from build123d import *

# Parameters (mm, degrees)
BOSS_EXTRUDE1_DEPTH = 5.772427301
SKETCH2_W           = 10.772427301
SKETCH2_H           = 33
BOSS_EXTRUDE2_DEPTH = 1
CUT_EXTRUDE1_DEPTH  = 2
SKETCH16_W          = 10.772427301
SKETCH16_H          = 1
BOSS_EXTRUDE4_DEPTH = 11
CUT_EXTRUDE2_REACH  = 24.797
SKETCH26_W          = 5
SKETCH26_H          = 10.722198916
CUT_EXTRUDE3_DEPTH  = 24.875254024
SKETCH13_W          = 3.772427301
SKETCH13_H          = 2.348567359
CUT_EXTRUDE4_DEPTH  = 1
SKETCH27_W          = 1
SKETCH27_H          = 12
BOSS_EXTRUDE5_DEPTH = 2.235
SKETCH28_W          = 1
SKETCH28_H          = 12
BOSS_EXTRUDE6_DEPTH = 2.235


with BuildPart() as part:
    # Sketch1 → Boss-Extrude1 (new body)
    with BuildSketch(Plane(origin=(6.659481674, 0, 0), x_dir=(0, 0, -1), z_dir=(1, 0, 0))):
        Polygon((-2.250948222, -1), (-2.966896165, -1), (-2.966896165, -2.348567359), align=None)
    extrude(amount=-BOSS_EXTRUDE1_DEPTH)

    # Sketch2 → Boss-Extrude2 (add)
    with BuildSketch(Plane(origin=(0, -1, 0), x_dir=(-1, 0, 0), z_dir=(0, 1, 0))):
        with Locations((-4.773268024, -2.096039546)):
            Rectangle(SKETCH2_W, SKETCH2_H)
        Polygon((-0.887054373, 2.966896165), (-0.887054373, 9.403960454), (-8.659481674, 9.403960454), (-8.659481674, -6.69042347), (-6.659481674, -6.69042347), (-6.659481674, 2.966896165), align=None, mode=Mode.SUBTRACT)
    extrude(amount=BOSS_EXTRUDE2_DEPTH)

    # Sketch7 → Cut-Extrude1 (cut)
    with BuildSketch(Plane.ZY.offset(-0.887054373)):
        Polygon((2.250948222, -1), (2.966896165, -2.348567359), (2.966896165, 0), (-6.69042347, 0), (-6.69042347, -1), align=None)
    extrude(amount=-CUT_EXTRUDE1_DEPTH, mode=Mode.SUBTRACT)

    # Sketch16 → Boss-Extrude4 (add)
    with BuildSketch(Plane(origin=(0, 0, 0), x_dir=(1, 0, 0), z_dir=(0, 1, 0))):
        with Locations((4.773268024, -13.903960454)):
            Rectangle(SKETCH16_W, SKETCH16_H)
    extrude(amount=BOSS_EXTRUDE4_DEPTH)

    # Sketch23 → Cut-Extrude2 (cut, up to next)
    with BuildSketch(Plane.ZY.offset(-2.887054373), mode=Mode.PRIVATE) as cut_extrude2_sk1:
        Polygon((2.250948222, 0), (2.250948222, -0.125928185), (3.122325521, -1.835650648), (3.712956794, -1.835650648), (3.712956794, 0), align=None)
    cut_extrude2_tool1 = extrude(cut_extrude2_sk1.sketch, amount=-CUT_EXTRUDE2_REACH, mode=Mode.PRIVATE) & part.part
    add(cut_extrude2_tool1.solids().sort_by_distance((2.887054, -0.784154, 3.151212))[0], mode=Mode.SUBTRACT)

    # Sketch26 → Cut-Extrude3 (cut, through all)
    with BuildSketch(Plane(origin=(0, 0, 0), x_dir=(1, 0, 0), z_dir=(0, 1, 0))):
        with Locations((4.772054373, 13.234940088)):
            Rectangle(SKETCH26_W, SKETCH26_H)
    extrude(amount=-CUT_EXTRUDE3_DEPTH, mode=Mode.SUBTRACT)

    # Sketch13 → Cut-Extrude4 (cut)
    with BuildSketch(Plane.XY.offset(2.966896165)):
        with Locations((4.773268024, -1.17428368)):
            Rectangle(SKETCH13_W, SKETCH13_H)
    extrude(amount=-CUT_EXTRUDE4_DEPTH, mode=Mode.SUBTRACT)

    # Sketch27 → Boss-Extrude5 (add)
    with BuildSketch(Plane.ZY.offset(0.612945627)):
        with Locations((13.903960454, 5)):
            Rectangle(SKETCH27_W, SKETCH27_H)
    extrude(amount=BOSS_EXTRUDE5_DEPTH)

    # Sketch28 → Boss-Extrude6 (add)
    with BuildSketch(Plane(origin=(10.159481674, 0, 0), x_dir=(0, 0, -1), z_dir=(1, 0, 0))):
        with Locations((-13.903960454, 5)):
            Rectangle(SKETCH28_W, SKETCH28_H)
    extrude(amount=BOSS_EXTRUDE6_DEPTH)


solid = part.part
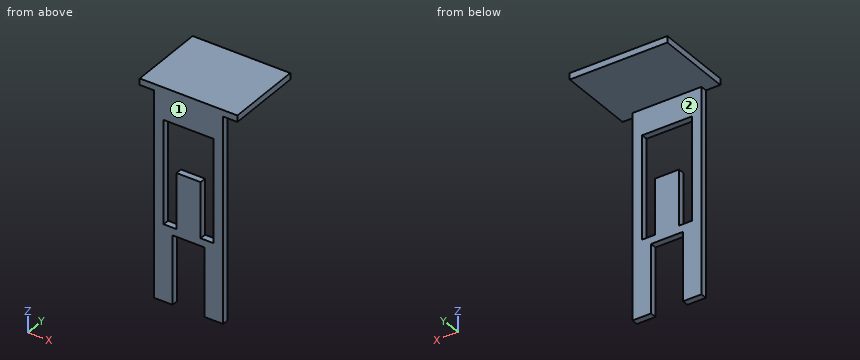
Read the model definition and answer for the solid it produces. Units are mm, in the model's axes. Face numbers are marked on the shaded views. A direction names the side the tool comes from. Coordinates: 2 decimals unless noted, no trailing zeros. Write each loop counter-clockwise with the first axis right and the second up, starting at its lowest first coordinate (ties: lowest second). Pieces come first, ordered by that corner, then holes. Notation, with made-up numbers: M 82,50 L 97,50 A26 cw 97,65 Z; hole C 33,12.25 d6. An arc over 180 degrees is marked long. Use a Markdown table: item, result.
Q1. The part is cut by section A-A, the plane x = 3.25. Write down the section's boundary in (y, z), then the cut area to 3 significant figures.
Answer block:
| item | result |
|---|---|
| outline | M -1,-7.87 L 0,-7.87 L 0,1.97 L -1,1.97 Z; M -1,9.4 L 0,9.4 L 0,13.4 L 11,13.4 L 11,14.4 L -1,14.4 Z |
| area | 25.8 mm2 |
Q2. Which of the six approach directions +Z, -Z, +X, -X, +Y, -Y give full straight-line access (tool end or side, diameter ignored) to the marked faces 1 and 2?
Answer block:
| item | result |
|---|---|
| face 1 | +Z, -Z, +X, -X, -Y |
| face 2 | -Z, +X, -X, +Y |
Q3. The part is cut by section B-B, the plane z = -3.5. Write down the section's boundary in (x, y).
Answer block:
| item | result |
|---|---|
| outline | M -0.61,-1 L 0.89,-1 L 0.89,0 L -0.61,0 Z; M 2.89,-1 L 6.66,-1 L 6.66,0 L 2.89,0 Z; M 8.66,-1 L 10.16,-1 L 10.16,0 L 8.66,0 Z |
Q4. Each of these flat-tipped pins is pushed along its axis until it touches: pin 1 Ø1.1 at (x, y) = (3.5, -0.5) entering from -Z; pin 2 Ø5 at (x, y) = (2, 8.5) entering from -Z; pin 3 Ø1.1 at (y, z) = (-0.5, -0.5) entering from +X; pin 4 Ø8 at (x, z) = (5.5, 7) entering from -Y. Where does it stop, or does it pass through?
Answer block:
| item | result |
|---|---|
| pin 1 | stops at z = -7.87 |
| pin 2 | stops at z = 13.4 |
| pin 3 | stops at x = 10.16 |
| pin 4 | stops at y = -1 |
Q5. Straight lines are drawn through the part: L1, parallel to Z at x = 3, y = 4; L2, parallel to Y at x = 0, z = -4. For each, find the intervals that lie inside material, in ascending order. Write a range as [from, to].
Answer block:
| item | result |
|---|---|
| L1 | z = [13.4, 14.4] |
| L2 | y = [-1, 0] |
Q6. The part is cut by section D-D, the plane y = 6.25. Write down the section's boundary in (x, z).
Answer block:
| item | result |
|---|---|
| outline | M -2.85,13.4 L 12.39,13.4 L 12.39,14.4 L -2.85,14.4 Z |
Q7. The part is cut by section C-C, the plane z = -15.5. Write down the section's boundary in (x, y), then the cut area to 3 significant figures.
Answer block:
| item | result |
|---|---|
| outline | M -0.61,-1 L 2.27,-1 L 2.27,0 L -0.61,0 Z; M 7.27,-1 L 10.16,-1 L 10.16,0 L 7.27,0 Z |
| area | 5.77 mm2 |
